Could you check a few things on this model? Use its own coordinates, in mm. Coordinates: 2 decimals unless noted, no trailing zeros. Write each loop counter-clockwise with the first axis right and the second up, starting at its lowest first coordinate (ties: lowest second). Pieces come first, ordered by that corner, then holes.
Item 1: For P1, Ø12, axis at y = -16.5, z = 30.5, coming from the +X side; P2, Ø5, axis at x = 28.5, y = -19.5, coming from the +Z side; P3, Ø3, axis at x = 3.5, y = -11, coming from the +Z side, each with a flat end and sliding along its axis, tell me the tip position at first contact or that it passes through.
Item 2: I want a section at A-A on x = 0. Please give me the cut outline in (y, z) (3 decimals).
Item 3: I want a section at B-B on z = 0. Please give me the cut outline in (x, y) (3 decimals).
Item 4: Thinking about a two-plate mould opening in Z: for faces 1 (the flat face through (-1, 0, 11)), 2 (the cylindrical face through (-11.012, -12.611, -49.592)), 3 (the cylindrical face through (-7.559, -12.878, -5.796)), which applies, +Z half, -Z half, draft (parallel to the pull), parting line (faces both ways), or undercut?
Item 5: I want a section at C-C on y = -13. Please give me the cut outline in (x, z) (3 decimals), then the cut area to 3 significant figures.
Item 6: If I drill on probe 1 along X at (y, z) = (-10.25, 5); probe 2 along X at (y, z) = (-16.5, 3.5); probe 3 along X at (y, z) = (-18.25, 26.5), over which ranges is the centre line in solid material (lowest first)?
from build123d import *

# Parameters (mm, degrees)
F0_R     = 50.8
F1_DEPTH = 25.4
F2_R     = 9.525
F3_DEPTH = 25.401
F4_R     = 6.35


with BuildPart() as f1:
    # F0 (on Front) → F1 (new body)
    with BuildSketch(Plane.XZ):
        Circle(F0_R)
    extrude(amount=F1_DEPTH)

    # F2 (on face) → F3 (cut, through all)
    with BuildSketch(Plane.XZ.offset(25.4)):
        Circle(F2_R)
    extrude(amount=-F3_DEPTH, mode=Mode.SUBTRACT)

    # F4
    f4_edges = [f1.edges().sort_by_distance(p)[0] for p in [
        (-50.8, -25.4, 0),
        (-50.8, 0, 0),
    ]]
    fillet(f4_edges, radius=F4_R)


solid = f1.part
Response values:
1. P1: stops at x = 44.5
1. P2: stops at z = 43.63
1. P3: stops at z = 50.76
2. outline: (-25.4, -44.45) arc R6.35 ccw to (-19.05, -50.8) - (-6.35, -50.8) arc R6.35 ccw to (0, -44.45) - (0, -9.525) - (-25.4, -9.525) - close; (-25.4, 9.525) - (0, 9.525) - (0, 44.45) arc R6.35 ccw to (-6.35, 50.8) - (-19.05, 50.8) arc R6.35 ccw to (-25.4, 44.45) - close
3. outline: (-50.8, -19.05) arc R6.35 ccw to (-44.45, -25.4) - (-9.525, -25.4) - (-9.525, 0) - (-44.45, 0) arc R6.35 ccw to (-50.8, -6.35) - close; (9.525, -25.4) - (44.45, -25.4) arc R6.35 ccw to (50.8, -19.05) - (50.8, -6.35) arc R6.35 ccw to (44.45, 0) - (9.525, 0) - close
4. face 1: draft
4. face 2: parting line
4. face 3: undercut
5. outline: circle Ø101.6 at (0, 0); hole circle Ø19.05 at (0, 0)
5. area: 7,820 mm2
6. probe 1: x = -50.55 to -8.11, 8.11 to 50.55
6. probe 2: x = -50.68 to -8.86, 8.86 to 50.68
6. probe 3: x = -43.34 to 43.34
